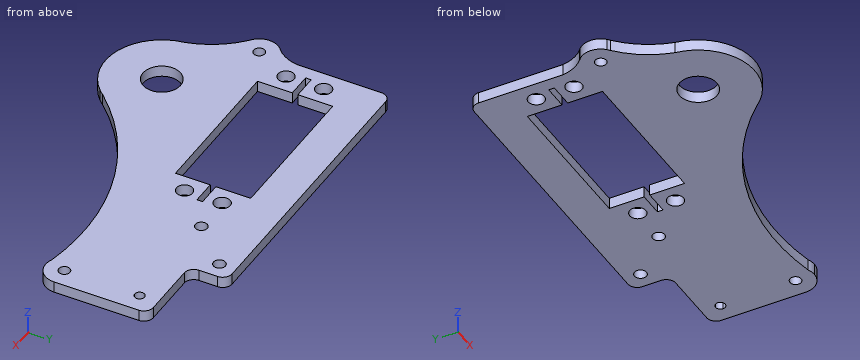
```python
from build123d import *

# Parameters (mm, degrees)
SKETCH_1_R          = 5
SKETCH_1_R_2        = 2.15
EXTRUDE_1_DEPTH     = 3
SKETCH_2_R          = 1.5
CUT_EXTRUDE_1_DEPTH = 117.657618697
CUT_EXTRUDE_3_DEPTH = 117.657618697
SKETCH_5_R          = 1.5
EXTRUDE_3_DEPTH     = 3
CUT_EXTRUDE_4_DEPTH = 117.657618697
SKETCH_7_R          = 1.6
CUT_EXTRUDE_6_DEPTH = 117.657618697
SKETCH_8_W          = 53
SKETCH_8_H          = 1.5
CUT_EXTRUDE_7_DEPTH = 117.657618697
SKETCH_9_W          = 79.9
SKETCH_9_H          = 10
SKETCH_9_R          = 1.6
EXTRUDE_4_DEPTH     = 3
FILLET_1_R          = 2.5


with BuildPart() as part:
    # ｽｹｯﾁ1 → ﾎﾞｽ - 押し出し1 (new body)
    with BuildSketch(Plane.XY):
        Polygon((10, 60), (0, 60), (0, 0), (100, 0), (100, 50), (100, 60), (50, 60), (50, 40), (10, 40), align=None)
        with Locations((20, 20)):
            Circle(SKETCH_1_R, mode=Mode.SUBTRACT)
        with Locations((5.25, 45)):
            Circle(SKETCH_1_R_2, mode=Mode.SUBTRACT)
        with Locations((5.25, 55)):
            Circle(SKETCH_1_R_2, mode=Mode.SUBTRACT)
        with Locations((54.75, 45)):
            Circle(SKETCH_1_R_2, mode=Mode.SUBTRACT)
        with Locations((54.75, 55)):
            Circle(SKETCH_1_R_2, mode=Mode.SUBTRACT)
    extrude(amount=EXTRUDE_1_DEPTH)

    # ｽｹｯﾁ2 → ｶｯﾄ - 押し出し1 (cut, through all)
    with BuildSketch(Plane.XY.offset(3)):
        with Locations((95, 35)):
            Circle(SKETCH_2_R)
    extrude(amount=-CUT_EXTRUDE_1_DEPTH, mode=Mode.SUBTRACT)

    # ｽｹｯﾁ4 → ｶｯﾄ - 押し出し3 (cut, through all)
    with BuildSketch(Plane.XY.offset(3)):
        with BuildLine():
            ThreePointArc((30.606601718, 9.393398282), (11.666446505, 7.527955815), (6.141807012, 25.740251485))
            ThreePointArc((6.141807012, 25.740251485), (5.992593584, 34.011854082), (1.731818145, 41.103219734))
            ThreePointArc((1.731818145, 41.103219734), (1.633577382, 41.194216579), (1.537689399, 41.287689399))
            ThreePointArc((1.537689399, 41.287689399), (0.399632454, 42.99091198), (0, 45))
            Line((0, 45), (0, 0))
            Line((0, 0), (100, 0))
            Line((100, 0), (100, 35))
            ThreePointArc((100, 35), (98.535533906, 31.464466094), (95, 30))
            ThreePointArc((95, 30), (93.906844507, 30.120962075), (92.866581158, 30.477995572))
            ThreePointArc((92.866581158, 30.477995572), (59.698938801, 28.658859349), (31.76111788, 10.689999666))
            ThreePointArc((31.76111788, 10.689999666), (31.202634234, 10.024981894), (30.606601718, 9.393398282))
        make_face()
    extrude(amount=-CUT_EXTRUDE_3_DEPTH, mode=Mode.SUBTRACT)

    # ｽｹｯﾁ5 → ﾎﾞｽ - 押し出し3 (add, through all)
    # profile 1 of 2: a face of its own
    with BuildSketch(Plane.XY.offset(3)):
        with BuildLine():
            ThreePointArc((-3.074339462, 38.943150628), (-3.301799792, 38.735793058), (-3.535533906, 38.535533906))
            ThreePointArc((-3.535533906, 38.535533906), (-5, 35), (-3.535533906, 31.464466094))
            ThreePointArc((-3.535533906, 31.464466094), (-3.171489153, 31.168816808), (-2.813054288, 30.866390733))
            ThreePointArc((-2.813054288, 30.866390733), (2.338239569, 30.580425844), (5, 35))
            ThreePointArc((5, 35), (2.194117441, 39.492866419), (-3.074339462, 38.943150628))
        make_face()
        with Locations((0, 35)):
            Circle(SKETCH_5_R, mode=Mode.SUBTRACT)
    # profile 2 of 2: a face of its own
    with BuildSketch(Plane.XY.offset(3)):
        with BuildLine():
            ThreePointArc((0, 45), (-1.007160055, 41.702552665), (-3.074339462, 38.943150628))
            ThreePointArc((-3.074339462, 38.943150628), (2.194117441, 39.492866419), (5, 35))
            ThreePointArc((5, 35), (2.338239569, 30.580425844), (-2.813054288, 30.866390733))
            ThreePointArc((-2.813054288, 30.866390733), (2.156646174, 25.048507639), (5.133931253, 18))
            ThreePointArc((5.133931253, 18), (5.125569714, 21.936833416), (6.141807012, 25.740251485))
            ThreePointArc((6.141807012, 25.740251485), (5.992593584, 34.011854082), (1.731818145, 41.103219734))
            ThreePointArc((1.731818145, 41.103219734), (0.4524509, 42.867859613), (0, 45))
        make_face()
    extrude(amount=-EXTRUDE_3_DEPTH)

    # ｽｹｯﾁ6 → ｶｯﾄ - 押し出し4 (cut, through all)
    with BuildSketch(Plane.XY.offset(3)):
        with BuildLine():
            ThreePointArc((96.3, 55), (95.919238816, 55.919238816), (95, 56.3))
            Line((95, 56.3), (95, 53.7))
            ThreePointArc((95, 53.7), (95.919238816, 54.080761184), (96.3, 55))
        make_face()
        with BuildLine():
            Line((95, 53.7), (95, 56.3))
            ThreePointArc((95, 56.3), (93.7, 55), (95, 53.7))
        make_face()
    extrude(amount=-CUT_EXTRUDE_4_DEPTH, mode=Mode.SUBTRACT)

    # ｽｹｯﾁ7 → ｶｯﾄ - 押し出し6 (cut, through all)
    with BuildSketch(Plane.XY.offset(3)):
        with Locations((64.9, 55)):
            Circle(SKETCH_7_R)
    extrude(amount=-CUT_EXTRUDE_6_DEPTH, mode=Mode.SUBTRACT)

    # ｽｹｯﾁ8 → ｶｯﾄ - 押し出し7 (cut, through all)
    with BuildSketch(Plane.XY.offset(3)):
        with Locations((30, 50)):
            Rectangle(SKETCH_8_W, SKETCH_8_H)
    extrude(amount=-CUT_EXTRUDE_7_DEPTH, mode=Mode.SUBTRACT)

    # ｽｹｯﾁ9 → ﾎﾞｽ - 押し出し4 (add, through all)
    with BuildSketch(Plane.XY.offset(3)):
        with Locations((39.95, 65)):
            Rectangle(SKETCH_9_W, SKETCH_9_H)
        with Locations((75.506601718, 65.606601718)):
            Circle(SKETCH_9_R, mode=Mode.SUBTRACT)
    extrude(amount=-EXTRUDE_4_DEPTH)

    # ﾌｨﾚｯﾄ1
    fillet_1_edges = [part.edges().sort_by_distance(p)[0] for p in [
        (0, 70, 1.5),
        (79.9, 70, 1.5),
        (79.9, 60, 1.5),
        (100, 60, 1.5),
    ]]
    fillet(fillet_1_edges, radius=FILLET_1_R)


solid = part.part
```
The model under review builds one solid part; all positions refer to its coordinate system, in mm. Give positions to 0.01 mm unless a question says otherwise; leave off trailing zeros. Loops run counter-clockwise (first coordinate to the right, second up) from the corner with the lowest first, then second, coordinate; pieces in that order, holes last. Notation, with made-up numbers: (40.25, 15) - (56.25, 15) arc R23 cw to (56.25, 40) - close; hole circle Ø4 at (12, 28). An arc over 180 degrees is marked (long way). Answer as a JSON object with one key per item and string values.
Q1. Insertion check: pin 1 (1.5 mm diameter, centred on x = 91, z = 1, fed in from +Y); pin 2 (8 mm diameter, centred on x = 20, y = 20, fed in from +Z); pin 3 (0.9 mm diameter, centred on x = 25.5, z = 1, fed in from -Y). Each pin has a flat end and moves straight along its axis. Give the tip position at first contact, or say it passes through.
Worked out:
{"pin 1": "stops at y = 60", "pin 2": "passes through", "pin 3": "stops at y = 5.88"}
Q2. Add section A-A on x = 20. State the section outline as (y, z) points, plus the area to 3 significant figures.
Worked out:
{"outline": "(5, 0) - (15, 0) - (15, 3) - (5, 3) - close; (25, 0) - (40, 0) - (40, 3) - (25, 3) - close; (60, 0) - (70, 0) - (70, 3) - (60, 3) - close", "area": "105 mm^2"}
Q3. Add section C-C on z = 2.55. Count the separate pieces of the cut face and the enclosed holes in it, plus the area to 3 significant figures.
Worked out:
{"separate pieces": "1", "enclosed holes": "11", "area": "3,680 mm^2"}
Q4. Add section B-B on x = 51. State the section outline as (y, z) points, plus the area to 3 significant figures.
Worked out:
{"outline": "(25.13, 0) - (49.25, 0) - (49.25, 3) - (25.13, 3) - close; (50.75, 0) - (70, 0) - (70, 3) - (50.75, 3) - close", "area": "130 mm^2"}
Q5. To check wall thickness, follow line 1 along Y through (x, z) = (15.5, 0.85); line 2 along Y through (x, z) = (18, 1.7); line 3 along X through (y, z) = (52.5, 1.1). State the ranges of each line that lie inside material, in increasing order.
Worked out:
{"line 1": "y = 5.69 to 17.82, 22.18 to 40, 60 to 70", "line 2": "y = 5.13 to 15.42, 24.58 to 40, 60 to 70", "line 3": "x = 0 to 10, 50 to 100"}
